Input: part model. Units: mm. Frame: model coordinates. Coordinates: 2 decimals unless noted, no trailing zeros. Loops run counter-clockwise (first coordinate to the right, second up) from the corner with the lowest first, then second, coordinate; pieces in that order, holes last. Notation, with made-up numbers: (21, 14) - (38, 14) arc R15 ccw to (38, 38) - close; hole circle Ø2 at (-19, 65). An arc over 180 degrees is marked (long way). Use a Markdown table: item, result. Add a question column.
1. Contact query for flat-ended pins moving along their axis: P1, Ø1, axis at x = -12, z = 193, coming from the -Y side; P2, Ø2.5, axis at x = 0.5, z = 636, coming from the +Y side; P3, Ø3.5, axis at y = -2.5, z = -61.5, coming from the +X side. Output: stop coordinate, or through.
2. Section query A-A on z = 587. Return the cut outline in (x, y).
3. Ray query, L1, parallel to Z at x = 2, y = 11.5; L2, parallel to Z at x = -3, y = 12; L3, parallel to X at y = 8.5, z = 577. Return the intervals inside material, ascending. Write a range as [from, to].
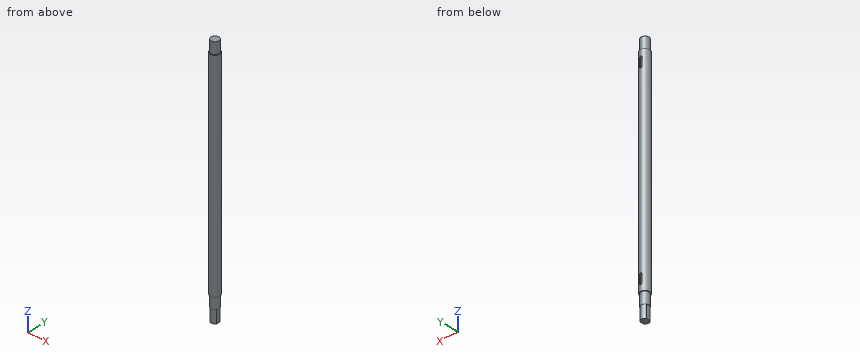
```python
from build123d import *

# Parameters (mm, degrees)
SKETCH1_R           = 15
BOSS_EXTRUDE1_DEPTH = 672
SKETCH2_R           = 12.5
BOSS_EXTRUDE3_DEPTH = 36
BOSS_EXTRUDE4_START = 90
SKETCH3_R           = 12.5
BOSS_EXTRUDE4_DEPTH = 90
SKETCH6_R           = 13.02430926
SKETCH6_R_2         = 12
CUT_EXTRUDE3_DEPTH  = 54
CUT_EXTRUDE2_DEPTH  = 4.5
MOVE_FACE1_BY       = 14
SKETCH7_W           = 4
SKETCH7_H           = 18
CUT_EXTRUDE4_DEPTH  = 40


with BuildPart() as part:
    # Sketch1 → Boss-Extrude1 (new body)
    with BuildSketch(Plane.XY):
        with Locations(Location((0, 0, 0), (0, 0, 180))):
            Circle(SKETCH1_R)
    extrude(amount=BOSS_EXTRUDE1_DEPTH)

    # Sketch2 → Boss-Extrude3 (add)
    with BuildSketch(Plane.XY.offset(672)):
        Circle(SKETCH2_R)
    extrude(amount=BOSS_EXTRUDE3_DEPTH)

    # Sketch3 → Boss-Extrude4 (add)
    with BuildSketch(Plane(origin=(0, 0, 0), x_dir=(-1, 0, 0), z_dir=(0, 0, -1)).offset(BOSS_EXTRUDE4_START)):
        with Locations(Location((0, 0, 0), (0, 0, 180))):
            Circle(SKETCH3_R)
    extrude(amount=-BOSS_EXTRUDE4_DEPTH)

    # Sketch6 → Cut-Extrude3 (cut)
    with BuildSketch(Plane(origin=(0, 0, -90), x_dir=(-1, 0, 0), z_dir=(0, 0, -1))):
        Circle(SKETCH6_R)
        Circle(SKETCH6_R_2, mode=Mode.SUBTRACT)
    extrude(amount=-CUT_EXTRUDE3_DEPTH, mode=Mode.SUBTRACT)

    # Sketch5 → Cut-Extrude2 (cut)
    with BuildSketch(Plane(origin=(0, 15, 0), x_dir=(1, 0, 0), z_dir=(0, 1, 0))):
        with BuildLine():
            Line((4, -624.5), (4, -649.5))
            ThreePointArc((4, -649.5), (0, -653.5), (-4, -649.5))
            Line((-4, -649.5), (-4, -624.5))
            ThreePointArc((-4, -624.5), (0, -620.5), (4, -624.5))
        make_face()
        with BuildLine():
            Line((4, -47.5), (4, -22.5))
            ThreePointArc((4, -22.5), (0, -18.5), (-4, -22.5))
            Line((-4, -22.5), (-4, -47.5))
            ThreePointArc((-4, -47.5), (0, -51.5), (4, -47.5))
        make_face()
    extrude(amount=-CUT_EXTRUDE2_DEPTH, mode=Mode.SUBTRACT)

    # Move Face1: a face moved inward by 14.0
    extrude(part.faces().sort_by_distance((0, 0, -90))[0], amount=MOVE_FACE1_BY, dir=(0, 0, 1), mode=Mode.SUBTRACT)

    # Sketch7 → Cut-Extrude4 (cut)
    with BuildSketch(Plane(origin=(0, 0, -76), x_dir=(-1, 0, 0), z_dir=(0, 0, -1))):
        with Locations((12.5, 0)):
            Rectangle(SKETCH7_W, SKETCH7_H)
        with Locations((-12.5, 0)):
            Rectangle(SKETCH7_W, SKETCH7_H)
    extrude(amount=-CUT_EXTRUDE4_DEPTH, mode=Mode.SUBTRACT)


solid = part.part
```
Resolved:
| question | item | result |
|---|---|---|
| 1 | P1 | y = -9.63 |
| 1 | P2 | y = 10.5 |
| 1 | P3 | x = 10.5 |
| 2 | outline | circle Ø30 at (0, 0) |
| 3 | L1 | [-76, 19.04], [50.96, 621.04], [652.96, 708] |
| 3 | L2 | [-36, 19.85], [50.15, 621.85], [652.15, 708] |
| 3 | L3 | [-12.36, 12.36] |
